Verification items for the finished model (mm, model axes). Face numbers are marked on the shaded views. A direction names the side the tool comes from. Round coordinates to 2 decimals unless told otherwise and drop trailing zeros. Order: outer loops, then holes, each group sorted by start corner. A loop starts at its lowest first (then second) coordinate and runs counter-clockwise, first axis right, second up. Notation, with made-up numbers: M -1.5,6.25 L 56.5,6.25 A27 ccw 56.5,44.25 Z; hole C 65,-29.75 d10. An arc over 180 degrees is marked long. Return JSON: item names as keys, results as strings. Group by question number.
from build123d import *

# Parameters (mm, degrees)
SKETCH1_R           = 34
BOSS_EXTRUDE1_DEPTH = 15
SKETCH2_R           = 48
BOSS_EXTRUDE2_DEPTH = 7.5
BOSS_EXTRUDE3_START = 7.5
SKETCH3_R           = 48
BOSS_EXTRUDE3_DEPTH = 7.5
SKETCH4_R           = 4
CUT_EXTRUDE1_DEPTH  = 30


with BuildPart() as part:
    # Sketch1 → Boss-Extrude1 (new body)
    with BuildSketch(Plane.XY):
        Circle(SKETCH1_R)
    extrude(amount=BOSS_EXTRUDE1_DEPTH)

    # Sketch2 → Boss-Extrude2 (add)
    with BuildSketch(Plane.XY.offset(15)):
        Circle(SKETCH2_R)
    extrude(amount=BOSS_EXTRUDE2_DEPTH)

    # Sketch3 → Boss-Extrude3 (add)
    with BuildSketch(Plane(origin=(0, 0, 0), x_dir=(-1, 0, 0), z_dir=(0, 0, -1)).offset(BOSS_EXTRUDE3_START)):
        with Locations(Location((0, 0, 0), (0, 0, 180))):
            Circle(SKETCH3_R)
    extrude(amount=-BOSS_EXTRUDE3_DEPTH)

    # Sketch4 → Cut-Extrude1 (cut)
    with BuildSketch(Plane(origin=(0, 0, -7.5), x_dir=(-1, 0, 0), z_dir=(0, 0, -1))):
        Circle(SKETCH4_R)
    extrude(amount=-CUT_EXTRUDE1_DEPTH, mode=Mode.SUBTRACT)


solid = part.part
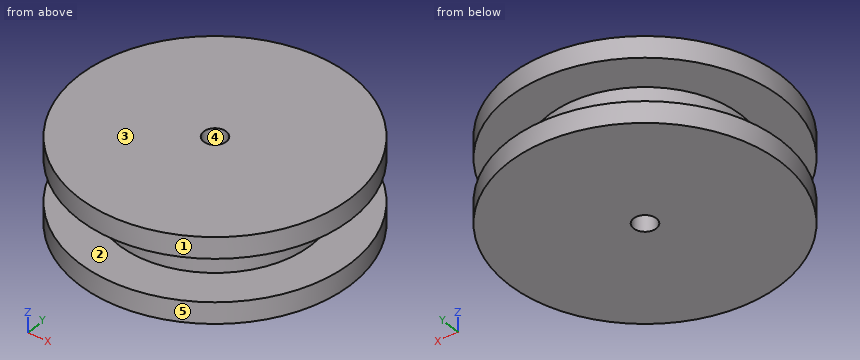
1. Cross-section at C-C (z = -4.25). Enter the section's corners in (x, y), plus the area to 3 significant figures.
2. Go/stop test with flat-tipped pins: pin 1 (6 mm diameter, centred on x = 4, z = 1, fed in from +Y); pin 2 (8 mm diameter, centred on x = 9.5, z = -2, fed in from -Y); pin 3 (3 mm diameter, centred on x = 4, z = -3, fed in from -Y). Record where each tip stops, or that it passes through.
3. Cross-section at A-A (y = 0). Enter the section's corners in (x, z), plus the area to 3 significant figures.
4. Cross-section at D-D (x = -23). Enter the section's corners in (y, z).
5. Draft check along Y on the marked faces 3, 4 and 5. Enter one of: +Y half, -Y half, draft (parallel to the pull), parting line (faces both ways), or undercut.
6. Access from +Z, -Z, +X, -X, +Y, -Y to the whole of each face (thin tool, end or side, straight path). Record for the marked faces 1 and 2.
7. Thickness scan on line 1 along Z through (x, y) = (-27, 32); line 2 along Y through (x, z) = (0, 4.25); line 3 along X through (y, z) = (-27, 12.25). Record the ranges inside material, lowest first. Write a range as from..to.
Computed:
{
 "1": {"outline": "C 0,0 d96; hole C 0,0 d8", "area": "7,190 mm²"},
 "2": {"pin 1": "stops at y = 47.99", "pin 2": "stops at y = -47.68", "pin 3": "stops at y = -47.93"},
 "3": {"outline": "M -48,-7.5 L -4,-7.5 L -4,22.5 L -48,22.5 L -48,15 L -34,15 L -34,0 L -48,0 Z; M 4,-7.5 L 48,-7.5 L 48,0 L 34,0 L 34,15 L 48,15 L 48,22.5 L 4,22.5 Z", "area": "2,220 mm²"},
 "4": {"outline": "M -42.13,-7.5 L 42.13,-7.5 L 42.13,0 L 25.04,0 L 25.04,15 L 42.13,15 L 42.13,22.5 L -42.13,22.5 L -42.13,15 L -25.04,15 L -25.04,0 L -42.13,0 Z"},
 "5": {"face 3": "draft", "face 4": "undercut", "face 5": "parting line"},
 "6": {"face 1": "+Z, -Z", "face 2": "none"},
 "7": {"line 1": "z = -7.5..0, 15..22.5", "line 2": "y = -34..-4, 4..34", "line 3": "x = -20.66..20.66"}
}
